The listing builds one solid part. Answer for the finished solid, in the listing's coordinates (mm). Coordinates: 2 decimals unless noted, no trailing zeros. Loops run counter-clockwise (first coordinate to the right, second up) from the corner with the lowest first, then second, coordinate; pieces in that order, holes last. Notation, with made-up numbers: (53, -4.5) -> (58, -4.5) arc R31 cw to (58, 28.5) -> close; hole circle Ø6 at (-35.75, 89.25). An arc over 180 degrees is marked (long way). Answer in a Markdown table with one row per item.
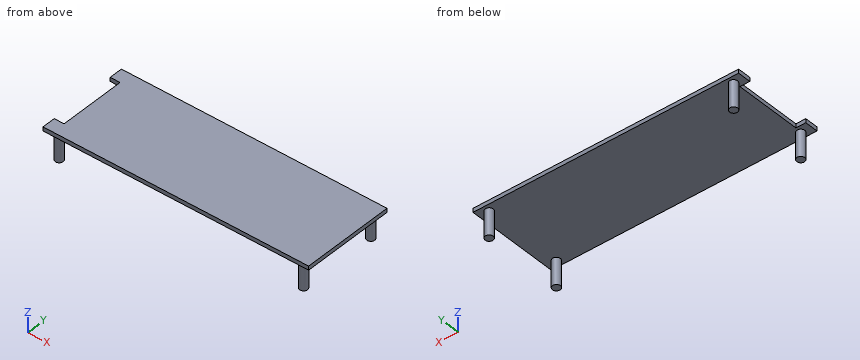
```python
from build123d import *

# Parameters (mm, degrees)
ESBO_O2_R                  = 3
RESSALTO_EXTRUS_O1_DEPTH   = 20
RESSALTO_EXTRUS_O1_2_DEPTH = 20
RESSALTO_EXTRUS_O1_3_DEPTH = 20
RESSALTO_EXTRUS_O1_4_DEPTH = 20
ESBO_O3_W                  = 200
ESBO_O3_H                  = 70
RESSALTO_EXTRUS_O2_DEPTH   = 3
ESBO_O4_W                  = 14.89887522
ESBO_O4_H                  = 50
CORTE_EXTRUS_O1_DEPTH      = 3


with BuildPart() as part:
    # Esbo_o2 → Ressalto-extrus_o1 (new body)
    with BuildSketch(Plane.XY):
        with Locations((192, -30)):
            Circle(ESBO_O2_R)
    extrude(amount=RESSALTO_EXTRUS_O1_DEPTH)



with BuildPart() as body_2:
    # Esbo_o2 → Ressalto-extrus_o1 2 (new body)
    with BuildSketch(Plane.XY):
        with Locations((192, 30)):
            Circle(ESBO_O2_R)
    extrude(amount=RESSALTO_EXTRUS_O1_2_DEPTH)


with BuildPart() as body_3:
    # Esbo_o2 → Ressalto-extrus_o1 3 (new body)
    with BuildSketch(Plane.XY):
        with Locations((8, 30)):
            Circle(ESBO_O2_R)
    extrude(amount=RESSALTO_EXTRUS_O1_3_DEPTH)


with BuildPart() as body_4:
    # Esbo_o2 → Ressalto-extrus_o1 4 (new body)
    with BuildSketch(Plane.XY):
        with Locations((8, -30)):
            Circle(ESBO_O2_R)
    extrude(amount=RESSALTO_EXTRUS_O1_4_DEPTH)


with BuildPart() as part_1:
    add(part.part)

    add(body_2.part)  # Ressalto-extrus_o2 merges body 2

    add(body_3.part)  # Ressalto-extrus_o2 merges body 3

    add(body_4.part)  # Ressalto-extrus_o2 merges body 4
    # Esbo_o3 → Ressalto-extrus_o2 (add)
    with BuildSketch(Plane.XY.offset(20)):
        with Locations((100, 0)):
            Rectangle(ESBO_O3_W, ESBO_O3_H)
    extrude(amount=RESSALTO_EXTRUS_O2_DEPTH)

    # Esbo_o4 → Corte-extrus_o1 (cut)
    with BuildSketch(Plane.XY.offset(23)):
        Rectangle(ESBO_O4_W, ESBO_O4_H)
    extrude(amount=-CORTE_EXTRUS_O1_DEPTH, mode=Mode.SUBTRACT)


solid = part_1.part
```
Item 1: Find the intervals of material crossed by probe 1 along Z at (x, y) = (50.5, -8); probe 2 along X at (y, z) = (4, 20.5); probe 3 along Y at (x, z) = (190.5, 6.75), in increasing order.
Findings below:
| item | result |
|---|---|
| probe 1 | z = 20 to 23 |
| probe 2 | x = 7.45 to 200 |
| probe 3 | y = -32.6 to -27.4, 27.4 to 32.6 |
Item 2: A cutting plane is placed at A-A, the plane y = 30. Determine the outline of the cut face in (x, z).
Findings below:
| item | result |
|---|---|
| outline | (0, 20) -> (5, 20) -> (5, 0) -> (11, 0) -> (11, 20) -> (189, 20) -> (189, 0) -> (195, 0) -> (195, 20) -> (200, 20) -> (200, 23) -> (0, 23) -> close |
Item 3: A cutting plane is placed at B-B, the plane z = 16.5. Determine the outline of the cut face in (x, y), plus the area to 3 significant figures.
Findings below:
| item | result |
|---|---|
| outline | circle Ø6 at (8, -30); circle Ø6 at (8, 30); circle Ø6 at (192, -30); circle Ø6 at (192, 30) |
| area | 113 mm2 |
Item 4: A cutting plane is placed at D-D, the plane x = 114. Determine the outline of the cut face in (y, z), plus the area to 3 significant figures.
Findings below:
| item | result |
|---|---|
| outline | (-35, 20) -> (35, 20) -> (35, 23) -> (-35, 23) -> close |
| area | 210 mm2 |
Item 5: A cutting plane is placed at C-C, the plane x = 192. Determine the outline of the cut face in (y, z).
Findings below:
| item | result |
|---|---|
| outline | (-35, 20) -> (-33, 20) -> (-33, 0) -> (-27, 0) -> (-27, 20) -> (27, 20) -> (27, 0) -> (33, 0) -> (33, 20) -> (35, 20) -> (35, 23) -> (-35, 23) -> close |
Item 6: Flat-ended cylindrical pins translate along their axes: pin 1 Ø6 at (x, y) = (37.5, 3) entering from -Z; pin 2 Ø8 at (y, z) = (23.5, 17) entering from +X; pin 3 Ø2 at (y, z) = (24.5, 18.5) entering from -X; pin 4 Ø0.9 at (y, z) = (-3.5, 21) entering from -X. Find the tip coordinate at first contact, or state that the pin passes through.
Findings below:
| item | result |
|---|---|
| pin 1 | stops at z = 20 |
| pin 2 | stops at x = 200 |
| pin 3 | passes through |
| pin 4 | stops at x = 7.45 |
